from build123d import *

# Parameters (mm, degrees)
SKETCH1_W           = 110
SKETCH1_H           = 225
BOSS_EXTRUDE1_DEPTH = 29
CUT_EXTRUDE1_REACH  = 130.539
CUT_EXTRUDE2_REACH  = 130.539
SKETCH4_R           = 8.5
CUT_EXTRUDE3_DEPTH  = 5
SKETCH5_R           = 10
CUT_EXTRUDE4_DEPTH  = 20
CUT_EXTRUDE5_REACH  = 130.539
SKETCH6_W           = 12
SKETCH6_H           = 11.5
M10_TAPPED_HOLE1_D  = 8.5
CUT_EXTRUDE6_REACH  = 130.539
SKETCH10_R          = 4


with BuildPart() as part:
    # Sketch1 → Boss-Extrude1 (new body)
    with BuildSketch(Plane(origin=(0, 0, 0), x_dir=(1, 0, 0), z_dir=(0, 1, 0))):
        Rectangle(SKETCH1_W, SKETCH1_H)
    extrude(amount=-BOSS_EXTRUDE1_DEPTH)

    # Sketch2 → Cut-Extrude1 (cut, up to next)
    with BuildSketch(Plane(origin=(0, 0, 0), x_dir=(1, 0, 0), z_dir=(0, 1, 0)), mode=Mode.PRIVATE) as cut_extrude1_sk1:
        with BuildLine():
            Line((-19, 37.36), (-19, 33.86))
            ThreePointArc((-19, 33.86), (-19.439339828, 32.799339828), (-20.5, 32.36))
            Line((-20.5, 32.36), (-34.5, 32.36))
            ThreePointArc((-34.5, 32.36), (-38.742640687, 30.602640687), (-40.5, 26.36))
            Line((-40.5, 26.36), (-40.5, -6.64))
            ThreePointArc((-40.5, -6.64), (-38.742640687, -10.882640687), (-34.5, -12.64))
            Line((-34.5, -12.64), (-20.5, -12.64))
            ThreePointArc((-20.5, -12.64), (-19.439339828, -13.079339828), (-19, -14.14))
            Line((-19, -14.14), (-19, -17.64))
            Line((-19, -17.64), (-42.5, -17.64))
            ThreePointArc((-42.5, -17.64), (-44.621320344, -16.761320344), (-45.5, -14.64))
            Line((-45.5, -14.64), (-45.5, 34.36))
            ThreePointArc((-45.5, 34.36), (-44.621320344, 36.481320344), (-42.5, 37.36))
            Line((-42.5, 37.36), (-19, 37.36))
        make_face()
    cut_extrude1_tool1 = extrude(cut_extrude1_sk1.sketch, amount=-CUT_EXTRUDE1_REACH, mode=Mode.PRIVATE) & part.part
    add(cut_extrude1_tool1.solids().sort_by_distance((-19.610512, 0, -35.61))[0], mode=Mode.SUBTRACT)

    # Sketch3 → Cut-Extrude2 (cut, up to next)
    with BuildSketch(Plane(origin=(0, 0, 0), x_dir=(1, 0, 0), z_dir=(0, 1, 0)), mode=Mode.PRIVATE) as cut_extrude2_sk1:
        with BuildLine():
            Line((19, 18.36), (31.5, 18.36))
            ThreePointArc((31.5, 18.36), (33.621320344, 17.481320344), (34.5, 15.36))
            Line((34.5, 15.36), (34.5, -10.64))
            ThreePointArc((34.5, -10.64), (33.621320344, -12.761320344), (31.5, -13.64))
            Line((31.5, -13.64), (19, -13.64))
            Line((19, -13.64), (19, -11.64))
            ThreePointArc((19, -11.64), (19.878679656, -9.518679656), (22, -8.64))
            Line((22, -8.64), (27.5, -8.64))
            ThreePointArc((27.5, -8.64), (28.914213562, -8.054213562), (29.5, -6.64))
            Line((29.5, -6.64), (29.5, 11.36))
            ThreePointArc((29.5, 11.36), (28.914213562, 12.774213562), (27.5, 13.36))
            Line((27.5, 13.36), (22, 13.36))
            ThreePointArc((22, 13.36), (19.878679656, 14.238679656), (19, 16.36))
            Line((19, 16.36), (19, 18.36))
        make_face()
    cut_extrude2_tool1 = extrude(cut_extrude2_sk1.sketch, amount=-CUT_EXTRUDE2_REACH, mode=Mode.PRIVATE) & part.part
    add(cut_extrude2_tool1.solids().sort_by_distance((25.25, 0, -18.004437))[0], mode=Mode.SUBTRACT)

    # Sketch4 → Cut-Extrude3 (cut)
    with BuildSketch(Plane.XZ.offset(29)):
        with Locations(Location((0, 100, 0), (0, 0, 270))):
            Circle(SKETCH4_R)
        with Locations(Location((0, -100, 0), (0, 0, 270))):
            Circle(SKETCH4_R)
    extrude(amount=-CUT_EXTRUDE3_DEPTH, mode=Mode.SUBTRACT)

    # Sketch5 → Cut-Extrude4 (cut)
    with BuildSketch(Plane(origin=(0, 0, 0), x_dir=(1, 0, 0), z_dir=(0, 1, 0))):
        with Locations(Location((-37.5, 72.36, 0), (0, 0, 270))):
            Circle(SKETCH5_R)
        with Locations(Location((-12.5, 72.36, 0), (0, 0, 270))):
            Circle(SKETCH5_R)
        with Locations(Location((12.5, 72.36, 0), (0, 0, 270))):
            Circle(SKETCH5_R)
        with Locations(Location((37.5, 72.36, 0), (0, 0, 270))):
            Circle(SKETCH5_R)
        with Locations(Location((37.5, -52.64, 0), (0, 0, 90))):
            Circle(SKETCH5_R)
        with Locations(Location((12.5, -52.64, 0), (0, 0, 90))):
            Circle(SKETCH5_R)
        with Locations(Location((-12.5, -52.64, 0), (0, 0, 90))):
            Circle(SKETCH5_R)
        with Locations(Location((-37.5, -52.64, 0), (0, 0, 90))):
            Circle(SKETCH5_R)
        with Locations(Location((0, 29.86, 0), (0, 0, 270))):
            Circle(SKETCH5_R)
        with Locations(Location((0, -10.14, 0), (0, 0, 270))):
            Circle(SKETCH5_R)
    extrude(amount=-CUT_EXTRUDE4_DEPTH, mode=Mode.SUBTRACT)

    # Sketch6 → Cut-Extrude5 (cut, up to next)
    with BuildSketch(Plane(origin=(0, 0, 0), x_dir=(1, 0, 0), z_dir=(0, 1, 0)), mode=Mode.PRIVATE) as cut_extrude5_sk1:
        with Locations((23.25, -106.75)):
            Rectangle(SKETCH6_W, SKETCH6_H)
    cut_extrude5_tool1 = extrude(cut_extrude5_sk1.sketch, amount=-CUT_EXTRUDE5_REACH, mode=Mode.PRIVATE) & part.part
    # Sketch6 → Cut-Extrude5 (cut, up to next)
    with BuildSketch(Plane(origin=(0, 0, 0), x_dir=(1, 0, 0), z_dir=(0, 1, 0)), mode=Mode.PRIVATE) as cut_extrude5_sk2:
        with Locations((-51.75, -106.75)):
            Rectangle(SKETCH6_W, SKETCH6_H)
    cut_extrude5_tool2 = extrude(cut_extrude5_sk2.sketch, amount=-CUT_EXTRUDE5_REACH, mode=Mode.PRIVATE) & part.part
    add(cut_extrude5_tool1.solids().sort_by_distance((23.25, 0, 106.75))[0], mode=Mode.SUBTRACT)
    add(cut_extrude5_tool2.solids().sort_by_distance((-51.75, 0, 106.75))[0], mode=Mode.SUBTRACT)

    # M10 Tapped Hole1 (through all)
    with Locations(Plane(origin=(0, 0, 0), x_dir=(1, 0, 0), z_dir=(0, 1, 0))):
        with Locations((-37.5, -72.64), (37.5, -72.64), (37.5, 92.36), (-37.5, 92.36)):
            Hole(M10_TAPPED_HOLE1_D / 2)

    # Sketch10 → Cut-Extrude6 (cut, up to next)
    with BuildSketch(Plane(origin=(0, 0, 0), x_dir=(1, 0, 0), z_dir=(0, 1, 0)), mode=Mode.PRIVATE) as cut_extrude6_sk1:
        with Locations(Location((0, 9.86, 0), (0, 0, 270))):
            Circle(SKETCH10_R)
    cut_extrude6_tool1 = extrude(cut_extrude6_sk1.sketch, amount=-CUT_EXTRUDE6_REACH, mode=Mode.PRIVATE) & part.part
    add(cut_extrude6_tool1.solids().sort_by_distance((0, 0, -9.86))[0], mode=Mode.SUBTRACT)

    # Cut-Sweep1: sweep along a path in Sketch12
    with BuildLine(Plane(origin=(0, 0, 0), x_dir=(1, 0, 0), z_dir=(0, 1, 0))) as cut_sweep1_path:
        Line((-19, 33.86), (-19, 37.36))
        Line((-19, 37.36), (-42.5, 37.36))
        ThreePointArc((-42.5, 37.36), (-44.621320344, 36.481320344), (-45.5, 34.36))
        Line((-45.5, 34.36), (-45.5, -14.64))
        ThreePointArc((-45.5, -14.64), (-44.621320344, -16.761320344), (-42.5, -17.64))
        Line((-42.5, -17.64), (-19, -17.64))
        Line((-19, -17.64), (-19, -14.14))
        ThreePointArc((-19, -14.14), (-19.439339828, -13.079339828), (-20.5, -12.64))
        Line((-20.5, -12.64), (-34.5, -12.64))
        ThreePointArc((-34.5, -12.64), (-38.742640687, -10.882640687), (-40.5, -6.64))
        Line((-40.5, -6.64), (-40.5, 26.36))
        ThreePointArc((-40.5, 26.36), (-38.742640687, 30.602640687), (-34.5, 32.36))
        Line((-34.5, 32.36), (-20.5, 32.36))
        ThreePointArc((-20.5, 32.36), (-19.439339828, 32.799339828), (-19, 33.86))
    # Sketch11 → Cut-Sweep1 (sweep, cut)
    with BuildSketch(Plane.XY):
        Polygon((-45.5, -24), (-45.5, 0), (-46.338098468, 0), align=None)
    sweep(path=cut_sweep1_path.line, transition=Transition.RIGHT, mode=Mode.SUBTRACT)

    # Cut-Sweep2: sweep along a path in Sketch14
    with BuildLine(Plane(origin=(0, 0, 0), x_dir=(1, 0, 0), z_dir=(0, 1, 0))) as cut_sweep2_path:
        Line((19, -11.64), (19, -13.64))
        Line((19, -13.64), (31.5, -13.64))
        ThreePointArc((31.5, -13.64), (33.621320344, -12.761320344), (34.5, -10.64))
        Line((34.5, -10.64), (34.5, 15.36))
        ThreePointArc((34.5, 15.36), (33.621320344, 17.481320344), (31.5, 18.36))
        Line((31.5, 18.36), (19, 18.36))
        Line((19, 18.36), (19, 16.36))
        ThreePointArc((19, 16.36), (19.878679656, 14.238679656), (22, 13.36))
        Line((22, 13.36), (27.5, 13.36))
        ThreePointArc((27.5, 13.36), (28.914213562, 12.774213562), (29.5, 11.36))
        Line((29.5, 11.36), (29.5, -6.64))
        ThreePointArc((29.5, -6.64), (28.914213562, -8.054213562), (27.5, -8.64))
        Line((27.5, -8.64), (22, -8.64))
        ThreePointArc((22, -8.64), (19.878679656, -9.518679656), (19, -11.64))
    # Sketch13 → Cut-Sweep2 (sweep, cut)
    with BuildSketch(Plane.XY):
        Polygon((34.5, -24), (34.5, 0), (35.338098468, 0), align=None)
    sweep(path=cut_sweep2_path.line, transition=Transition.RIGHT, mode=Mode.SUBTRACT)


solid = part.part
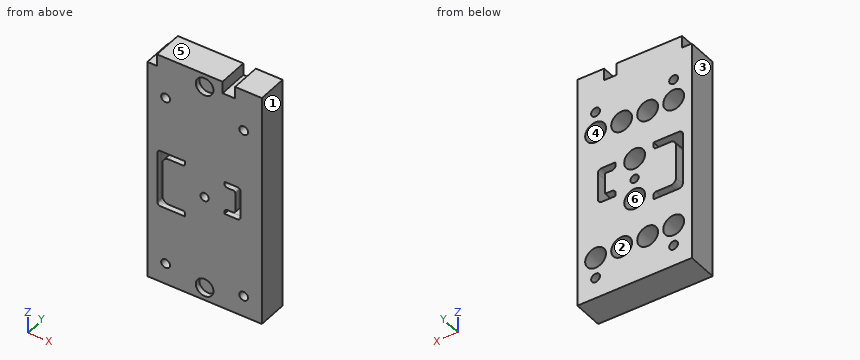
CAD build for the part. Positions are in the model's coordinates, mm. Face numbers are marked on the shaded views. A direction names the side the tool comes from. Give positions to 0.01 mm unless a question says otherwise; leave off trailing zeros. Write each loop counter-clockwise with the first axis right and the second up, starting at its lowest first coordinate (ties: lowest second). Pieces come first, ordered by that corner, then holes. Notation, with made-up numbers: (66, -10) - (82, -10) arc R16 ccw to (82, 6) - close; hole circle Ø10 at (-27.5, -1.5). An arc over 180 degrees is marked (long way). Answer as CSV lines item,"result".
Q1. Band-saw the part on B-B (z = 72.64). Give the cut face in (x, y), and give its area (3 significant figures).
Result set:
outline,"(-55, -29) - (-41.75, -29) - (-41.75, 0) - (-55, 0) - close; (-33.25, -29) - (33.25, -29) - (33.25, 0) - (-33.25, 0) - close; (41.75, -29) - (55, -29) - (55, 0) - (41.75, 0) - close"
area,"2,700 mm²"
Q2. Band-saw the part on C-C (x = -12.5). Give the cut face in (y, z), and give its area (4 significant figures).
Result set:
outline,"(-29, -112.5) - (0, -112.5) - (0, -82.36) - (-20, -82.36) - (-20, -62.36) - (0, -62.36) - (0, 42.64) - (-20, 42.64) - (-20, 62.64) - (0, 62.64) - (0, 112.5) - (-29, 112.5) - close"
area,"5,725 mm²"
Q3. 3-axis set-ups, long thin cutter, end or side, ignore diameter. For the marked faces 1 and 2: which of +Z, -Z, +X, -X, +Y, -Y reach the whole face in a straight line?
Result set:
face 1,"+Z, -Z, +X, +Y, -Y"
face 2,"+Y"
Q4. Drill centre lines: line 1 (X direction, y = -7.75, z = 53.5); line 2 (X direction, y = -14.5, z = 72.64); line 3 (Z direction, x = 37.5, y = -20.5). Where is each one in solid material? Low to high. Write a range as from..to.
Result set:
line 1,"-55..-47.46, -27.54..-22.46, -2.54..2.54, 22.46..27.54, 47.46..55"
line 2,"-55..-41.75, -33.25..33.25, 41.75..55"
line 3,"-112.5..-96.61, -88.11..68.39, 76.89..112.5"
Q5. Flat gauge pins, fed straight in: pin 1 Ø12.5 at (y, z) = (-15.5, 107.5) entering from -X; pin 2 Ø16 at (x, z) = (-14, 53) entering from +Y; pin 3 Ø22 at (x, z) = (-32.5, -74.5) entering from +Y; pin 4 Ø8.5 at (x, z) = (3, -102.5) entering from -Y. Where does each tip first touch, or does it go through?
Result set:
pin 1,"x = -45.75"
pin 2,"y = -20"
pin 3,"y = 0"
pin 4,"y = -24"
Q6. Pull direction X, two halves, no side cores. Call the marked faces 3, 4, 5 and 6: released by +X, released by -X, zero draft, split by the parting line, or undercut.
Result set:
face 3,"released by -X"
face 4,"undercut"
face 5,"zero draft"
face 6,"undercut"
Q7. Band-saw the part on D-D (z = -24). Give the cut face in (x, y).
Result set:
outline,"(-55, -29) - (-45.5, -29) - (-45.5, -24) - (-46.34, 0) - (-55, 0) - close; (-40.5, -29) - (55, -29) - (55, 0) - (8.1, 0) - (8.1, -20) - (-8.1, -20) - (-8.1, 0) - (-39.66, 0) - (-40.5, -24) - close"
Q8. Band-saw the part on A-A (x = 37.5). Give the cut face in (y, z), and give its area (3 significant figures).
Result set:
outline,"(-29, -112.5) - (0, -112.5) - (0, -96.61) - (-29, -96.61) - close; (-29, -88.11) - (0, -88.11) - (0, -82.36) - (-20, -82.36) - (-20, -62.36) - (0, -62.36) - (0, 42.64) - (-20, 42.64) - (-20, 62.64) - (0, 62.64) - (0, 68.39) - (-29, 68.39) - close; (-29, 76.89) - (0, 76.89) - (0, 112.5) - (-29, 112.5) - close"
area,"5,230 mm²"
